Source: CAD feature listing. Evaluate the final solid. Frame: model axes, mm. Face numbers are marked on the shaded views. A direction names the side the tool comes from. Give positions to 0.01 mm unless a question says otherwise; leave off trailing zeros. Order: outer loops, then holes, each group sorted by start corner. A loop starts at its lowest first (then second) coordinate and runs counter-clockwise, first axis right, second up.
1) Access query for the marked faces 5 and 6. Directions: +Z, -Z, +X, -X, +Y, -Y. A direction counts if a zero-diameter tool reaches every point of the face in a straight line with its end or side. Return the directions, or none.
2) First-contact query: P1, Ø1, axis at x = 7, y = -13, coming from the -Z side; P2, Ø14.5, axis at x = -1, y = -10, coming from the -Z side; P3, Ø5, axis at y = -20.5, z = 0, coming from the +X side; P4, Ø4, axis at x = 18, y = -23.5, coming from the -Z side. Flat tips, straight axial feed; report the tip coordinate or a pass-through.
3) Material intervals for line 1 (Y direction, x = 0, z = -12.25); line 2 (Z direction, x = 6, y = 11.5); line 3 (Z direction, x = 5.5, y = 4.5), sorted ascending.
4) Draft query along Y for the marked faces 1, 2, 3 and 4. Return one class per face: released by +Y, released by -Y, zero draft, split by the parting line, or undercut.
5) Section D-D, the plane y = 22. Return loops of the section in (x, z).
6) Section C-C, the plane z = -13.75. Return loops of the section in (x, y), plus the area to 3 significant figures.
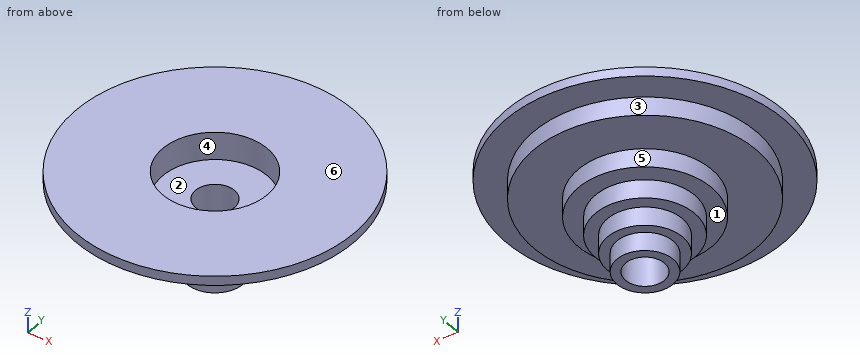
Autodesk Inventor part; units mm, degrees
ref_plane "YZ Plane" through (0, 0, 0) normal (1, 0, 0) x (0, 1, 0)
ref_plane "XZ Plane" through (0, 0, 0) normal (0, 1, 0) x (-1, 0, 0)
ref_plane "XY Plane" through (0, 0, 0) normal (0, 0, 1) x (1, 0, 0)
sketch "Sketch1" plane through (0, 0, 0) normal (0, 0, 1) x (1, 0, 0)
  circle A0 centre (0, 0) radius 11.3
  circle A1 centre (0, 0) radius 30
  dimension "d0" = 22.6
  dimension "d1" = 60
extrude "Extrusion1" add sketch "Sketch1" along normal blind 6
sketch "Sketch2" plane through (0, 0, 0) normal (1, 0, 0) x (0, 1, 0)
  line L0 (-30, 0) -> (30, 0)
  line L1 (0, 0) -> (0, -22.2563)
  line L2 (0, -28.8) -> (0, 4.8)
  line L3 (20.103, -4) -> (-2.6994, -4) construction
  line L4 (20.103, -8) -> (-2.6994, -8) construction
  line L5 (20.103, -12) -> (-2.6994, -12) construction
  line L6 (20.103, -16) -> (-2.6994, -16) construction
  line L7 (20.103, -20) -> (-2.6994, -20) construction
  line L8 (20.103, -24) -> (-2.6994, -24) construction
  line L9 (10.7198, -8) -> (10.7198, -4)
  line L10 (14.402, -4) -> (10.7198, -4)
  line L11 (8.1057, -12) -> (8.1057, -8)
  line L12 (10.7198, -8) -> (8.1057, -8)
  line L13 (6.0862, -16) -> (6.0862, -12)
  line L14 (8.1057, -12) -> (6.0862, -12)
  line L15 (6.0862, -16) -> (4.4759, -16)
  line L16 (14.402, -4) -> (14.402, 0)
  line L17 (4.4759, -16) -> (0, -16)
  point P0 (0, -11.3553)
  point P1 (0, -24)
  point P2 (0, -20)
  dimension "d8" = 4
  dimension "d11" = 4
revolve "Revolution1" add sketch "Sketch2" angle 360 about axis through (0, 0, -10) along (0, 0, 1)
sketch "Sketch3" plane through (0, 0, 0) normal (0, 0, 1) x (1, 0, 0)
  circle A0 centre (0, 0) radius 4.2
  dimension "d5" = 8.4
extrude "Extrusion2" cut sketch "Sketch3" against normal through all
sketch "Sketch4" plane through (0, 0, 0) normal (0, 0, -1) x (-1, 0, 0)
  circle A0 centre (0, 0) radius 24
  circle A1 centre (0, 0) radius 30
  dimension "d16" = 48
extrude "Extrusion3" cut sketch "Sketch4" against normal blind 4
properties part number "spool diam support"
From the geometry:
1. face 5: -Z
1. face 6: +Z, +X, -X, +Y, -Y
2. P1: stops at z = -4
2. P2: stops at z = -16
2. P3: stops at x = 15.87
2. P4: stops at z = 4
3. line 1: y = -6.09 to -4.2, 4.2 to 6.09
3. line 2: z = -4 to 6
3. line 3: z = -12 to 0
4. face 1: zero draft
4. face 2: undercut
4. face 3: split by the parting line
4. face 4: undercut
5. outline: (-20.4, 4) - (-9.59, 4) - (-9.59, 0) - (9.59, 0) - (9.59, 4) - (20.4, 4) - (20.4, 6) - (-20.4, 6) - close
6. outline: circle Ø12.17 at (0, 0); hole circle Ø8.4 at (0, 0)
6. area: 61.0 mm2
